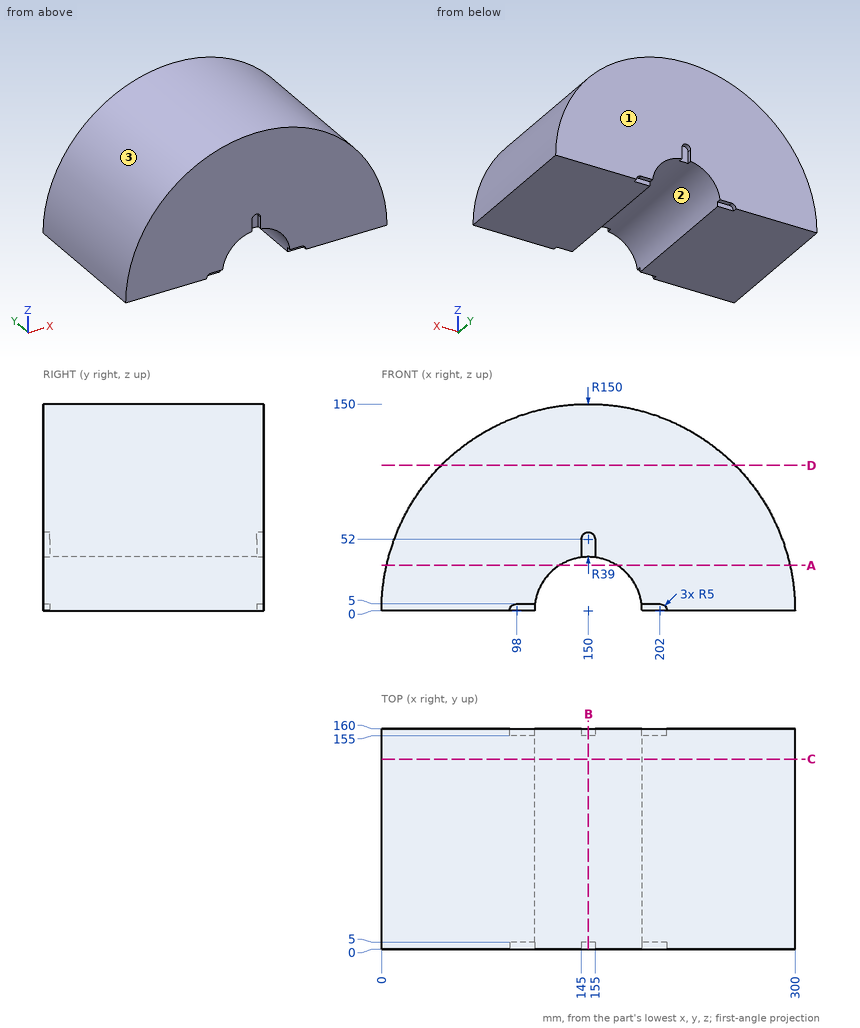
Can you work these out from the drawing? Everything is in mm from the part's minimum corner. Give positions to 0.01 mm unless a question says otherwise; leave off trailing zeros. Order: outer loops, then holes, each group sorted by start corner. A loop starts at its lowest first (then second) coordinate and runs counter-clockwise, first axis right, second up. Notation, with made-up numbers: M 54,34.25 L 107,34.25 A10 cw 107,40.25 Z; hole C -31.75,72 d10. An arc over 180 degrees is marked long. Write item = value, one per line. Start each with the question number.
Q1. I need wall thicknesses on probe 1 along X at (y, z) = (113, 22.5); probe 2 along X at (y, z) = (135.5, 25); probe 3 along Z at (x, y) = (23.5, 112). Which ranges of each line are inside material? Lowest first, please. Write a range as [from, to].
Q2. Will these pins go through, and if not, where does the flat tip stop? pin 1 Ø4 at (y, z) = (157.5, 43) entering from -X; pin 2 Ø1.5 at (x, z) = (102, 3) entering from +Y; pin 3 Ø6 at (x, y) = (209, 47) entering from +Z; pin 4 Ø2 at (x, z) = (199, 128) entering from -Y.
Q3. Suppose I cut it at B-B (x = 150). Write out the boundary of the cut face in (y, z), plus the area to 3 significant figures.
Q4. We'd pull the mould along X, two halves only. Please class the marked faces 1, 2 and 3: pulls with the +X half, pulls with the -X half, needs draft (parallel to the pull), parting line crosses it, or undercut.
Q5. Suppose I cut it at A-A (z = 33). Write out the boundary of the cut face in (x, y).
Q6. Suppose I cut it at D-D (z = 105.5). Write out the boundary of the cut face in (x, y), plus the area to 3 significant figures.
Q7. Suppose I cut it at C-C (y = 138). Write out the boundary of the cut face in (x, z), plus the area to 3 significant figures.
Check result:
q1.probe_1 = [1.7, 118.14], [181.86, 298.3]
q1.probe_2 = [2.1, 120.07], [179.93, 297.9]
q1.probe_3 = [0, 80.61]
q2.pin_1 = 5.71
q2.pin_2 = 155
q2.pin_3 = 139.15
q2.pin_4 = 0
q3.outline = M 0,57 L 5,57 L 5,39 L 155,39 L 155,57 L 160,57 L 160,150 L 0,150 Z
q3.area = 17,600 mm2
q4.face_1 = needs draft
q4.face_2 = undercut
q4.face_3 = parting line crosses it
q5.outline = M 3.68,0 L 129.22,0 L 129.22,160 L 3.68,160 Z; M 170.78,0 L 296.32,0 L 296.32,160 L 170.78,160 Z
q6.outline = M 43.37,0 L 256.63,0 L 256.63,160 L 43.37,160 Z
q6.area = 34,100 mm2
q7.outline = M 0,0 L 111,0 A39 cw 189,0 L 300,0 A150 ccw Z
q7.area = 33,000 mm2
